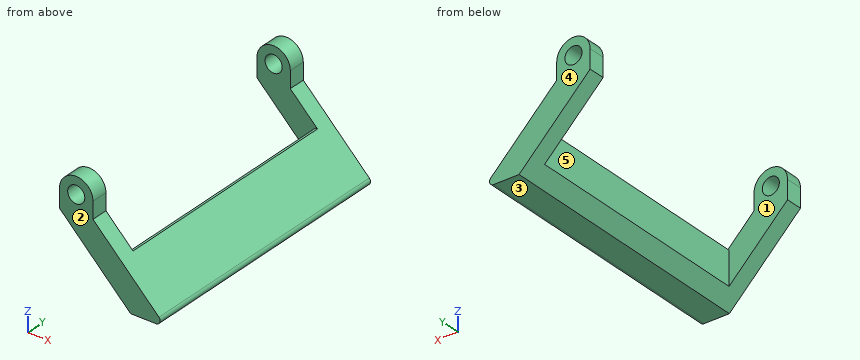
from build123d import *

# Parameters (mm, degrees)
BOSS_EXTRUDE1_DEPTH            = 4.00000003
BOSS_EXTRUDE2_DEPTH            = 56.99999997
BOSS_EXTRUDE3_DEPTH            = 4
F_4_1_4_1_DIAMETER_HOLE1_D     = 4.1
F_4_1_4_1_DIAMETER_HOLE1_DEPTH = 4
F_4_1_4_1_DIAMETER_HOLE2_D     = 4.1
F_4_1_4_1_DIAMETER_HOLE2_DEPTH = 65


with BuildPart() as part:
    # Sketch1 → Boss-Extrude1 (new body)
    with BuildSketch(Plane.XZ.offset(61.6)):
        with BuildLine():
            Line((-25.5, 17.014718626), (-8.485281374, 0))
            Line((-8.485281374, 0), (-2.414213562, 0))
            ThreePointArc((-2.414213562, 0), (-1.49033403, 0.617316568), (-1.707106781, 1.707106781))
            Line((-1.707106781, 1.707106781), (-17.5, 17.5))
            Line((-17.5, 17.5), (-17.5, 21.5))
            ThreePointArc((-17.5, 21.5), (-21.5, 25.5), (-25.5, 21.5))
            Line((-25.5, 21.5), (-25.5, 17.014718626))
        make_face()
    extrude(amount=-BOSS_EXTRUDE1_DEPTH)

    # Sketch2 → Boss-Extrude2 (add)
    with BuildSketch(Plane(origin=(0, -57.59999997, 0), x_dir=(-1, 0, 0), z_dir=(0, 1, 0))):
        with BuildLine():
            Line((1.707106781, 1.707106781), (11.000000003, 11.000000003))
            Line((11.000000003, 11.000000003), (11.500000002, 11.000000003))
            Line((11.500000002, 11.000000003), (11.500000002, 3.014718628))
            Line((11.500000002, 3.014718628), (8.485281374, 0))
            Line((8.485281374, 0), (2.414213562, 0))
            ThreePointArc((2.414213562, 0), (1.49033403, 0.617316568), (1.707106781, 1.707106781))
        make_face()
    extrude(amount=BOSS_EXTRUDE2_DEPTH)

    # Sketch3 → Boss-Extrude3 (add)
    with BuildSketch(Plane(origin=(0, -0.6, 0), x_dir=(-1, 0, 0), z_dir=(0, 1, 0))):
        with BuildLine():
            Line((8.485281374, 0), (2.414213562, 0))
            ThreePointArc((2.414213562, 0), (1.49033403, 0.617316568), (1.707106781, 1.707106781))
            Line((1.707106781, 1.707106781), (17.500000001, 17.500000001))
            Line((17.500000001, 17.500000001), (17.500000001, 21.5))
            ThreePointArc((17.500000001, 21.5), (21.500000001, 25.5), (25.5, 21.5))
            Line((25.5, 21.5), (25.5, 17.014718626))
            Line((25.5, 17.014718626), (8.485281374, 0))
        make_face()
    extrude(amount=BOSS_EXTRUDE3_DEPTH)

    # Ø4.1 (4.1) Diameter Hole1
    with Locations(Plane(origin=(0, 3.4, 0), x_dir=(1, 0, 0), z_dir=(0, 1, 0))):
        with Locations((-21.5, -21.5)):
            Hole(F_4_1_4_1_DIAMETER_HOLE1_D / 2, depth=F_4_1_4_1_DIAMETER_HOLE1_DEPTH)

    # Ø4.1 (4.1) Diameter Hole2
    with Locations(Plane(origin=(0, -61.6, 0), x_dir=(-1, 0, 0), z_dir=(0, -1, 0))):
        with Locations((21.5, -21.5)):
            Hole(F_4_1_4_1_DIAMETER_HOLE2_D / 2, depth=F_4_1_4_1_DIAMETER_HOLE2_DEPTH)


solid = part.part
Design review of the part built by this model. Coordinates are the model's own, in mm. Face numbers are marked on the shaded views. A direction names the side the tool comes from. Coordinates: 2 decimals unless noted, no trailing zeros. Order: outer loops, then holes, each group sorted by start corner. A loop starts at its lowest first (then second) coordinate and runs counter-clockwise, first axis right, second up.
Item 1: For line 1 (Y direction, x = -16.5, z = 15.25); line 2 (X direction, y = 0.7, z = 21.5); line 3 (Z direction, x = -21.5, y = -60.2), list the stretches that pass through material, from the lowest coordinate up.
Item 2: Take a section at C-C, the plane x = -21.5. Write out the cut boundary in (y, z).
Item 3: Take a section at D-D, the plane y = -49.5. Write out the cut boundary in (x, z), then the cut area to 3 significant figures.
Item 4: For the marked faces 1 and 2, list the 3-axis set-ups (+Z, -Z, +X, -X, +Y, -Y) from which the entire face can be reached by the end or side of a thin tool; tool diameter is ignored.
Item 5: For pin 1 Ø2.5 at (y, z) = (-27, 5) entering from -X; pin 2 Ø2 at (y, z) = (-12, 9.5) entering from +X; pin 3 Ø8 at (x, y) = (-12.5, -20.5) entering from +Z; pin 4 Ø3.5 at (x, z) = (-21.5, 21.5) entering from -Y, all flat-tipped, find the tip position at first contact; note any pin that passes through.
Item 6: Take a section at B-B, the plane x = -14.25. Write out the cut boundary in (y, z), then the cut area to 3 significant figures.
Item 7: The part is to be moulded in two halves that separate along Y. For the marked faces 3, 4 and 5, say which applies: pulls with the +Y half, pulls with the -Y half, needs draft (parallel to the pull), parting line crosses it, or undercut.
Item 8: Take a section at A-A, the plane z = 15.25. Write out the cut boundary in (x, y).
The answers:
1. line 1: y = -61.6 to -57.6, -0.6 to 3.4
1. line 2: x = -25.5 to -23.55, -19.45 to -17.5
1. line 3: z = 13.01 to 19.45, 23.55 to 25.5
2. outline: (-61.6, 13.01) - (-57.6, 13.01) - (-57.6, 19.45) - (-61.6, 19.45) - close; (-61.6, 23.55) - (-57.6, 23.55) - (-57.6, 25.5) - (-61.6, 25.5) - close; (-0.6, 13.01) - (3.4, 13.01) - (3.4, 19.45) - (-0.6, 19.45) - close; (-0.6, 23.55) - (3.4, 23.55) - (3.4, 25.5) - (-0.6, 25.5) - close
3. outline: (-11.5, 3.01) - (-8.49, 0) - (-2.41, 0) arc R1 ccw to (-1.71, 1.71) - (-11, 11) - (-11.5, 11) - close
3. area: 60.2 mm2
4. face 1: +Z, -Z, -X
4. face 2: +Z, -Z, +X, -X, -Y
5. pin 1: stops at x = -11.5
5. pin 2: stops at x = -8.5
5. pin 3: stops at z = 11
5. pin 4: passes through
6. outline: (-61.6, 5.76) - (-57.6, 5.76) - (-57.6, 14.25) - (-61.6, 14.25) - close; (-0.6, 5.76) - (3.4, 5.76) - (3.4, 14.25) - (-0.6, 14.25) - close
6. area: 67.9 mm2
7. face 3: needs draft
7. face 4: pulls with the +Y half
7. face 5: undercut
8. outline: (-23.74, -61.6) - (-15.25, -61.6) - (-15.25, -57.6) - (-23.74, -57.6) - close; (-23.74, -0.6) - (-15.25, -0.6) - (-15.25, 3.4) - (-23.74, 3.4) - close
